from build123d import *

# Parameters (mm, degrees)
SKETCH1_R           = 74.5
BOSS_EXTRUDE1_DEPTH = 385.699
SKETCH2_W           = 27.8577878
SKETCH2_H           = 360.299
SKETCH3_R           = 4.499991
CUT_EXTRUDE1_DEPTH  = 400.830237227
CIRPATTERN1_COUNT   = 4
FILLET1_R           = 10


with BuildPart() as part:
    # Sketch1 → Boss-Extrude1 (new body)
    with BuildSketch(Plane(origin=(0, 0, 0), x_dir=(1, 0, 0), z_dir=(0, 1, 0))):
        with Locations(Location((0, 0, 0), (0, 0, 270))):
            Circle(SKETCH1_R)
    extrude(amount=BOSS_EXTRUDE1_DEPTH)

    # Sketch2 → Cut-Revolve4 (revolve, cut)
    with BuildSketch(Plane.XY, mode=Mode.PRIVATE) as cut_revolve4_sk:
        with Locations((-60.5711061, 192.8495)):
            Rectangle(SKETCH2_W, SKETCH2_H)
    revolve(cut_revolve4_sk.sketch.rotate(Axis((0, 385.699, 0), (0, -1, 0)), 270), axis=Axis((0, 385.699, 0), (0, -1, 0)), mode=Mode.SUBTRACT)

    # Sketch3 → Cut-Extrude1 (cut, through all)
    with BuildSketch(Plane.XZ):
        with Locations(Location((0, 66.000122, 0), (0, 0, 270))):
            Circle(SKETCH3_R)
    cut_extrude1 = extrude(amount=-CUT_EXTRUDE1_DEPTH, mode=Mode.SUBTRACT)

    # CirPattern1: Cut-Extrude1 ×4 about axis
    cirpattern1_axis = Axis((0, 0, 0), (0, 1, 0))
    for i in range(1, CIRPATTERN1_COUNT):
        add(cut_extrude1.rotate(cirpattern1_axis, i * 360 / CIRPATTERN1_COUNT), mode=Mode.SUBTRACT)

    # Fillet1
    fillet1_edges = [part.edges().sort_by_distance(p)[0] for p in [
        (0, 12.7, -46.6422122),
        (0, 372.999, -46.6422122),
    ]]
    fillet(fillet1_edges, radius=FILLET1_R)


solid = part.part
The listing builds one solid part. Answer for the finished solid, in the listing's coordinates (mm). A direction names the side the tool comes from. Coordinates: 2 decimals unless noted, no trailing zeros. Order: outer loops, then holes, each group sorted by start corner. A loop starts at its lowest first (then second) coordinate and runs counter-clockwise, first axis right, second up. Notation, with made-up numbers: (-8, 31) -> (-4, 31) arc R17 cw to (-4, 40) -> close; hole circle Ø10 at (76, -7). An arc over 180 degrees is marked (long way). Answer in a Markdown table with one row per item. Add a question column.
Item 1: Find section A-A (x = 0). State how many separate pieces and enclosed holes the cut face has, then the cut area to 3 significant figures.
Item 2: Find the intervals of material crossed by L1, parallel to Y at x = -39.5, z = -48; L2, parallel to Y at x = 17, z = 46; L3, parallel to X at y = 195.5, z = 24.5, in increasing order. Write a range as from..to.
Item 3: Each of these flat-tipped pins is pushed along its axis until it touches: P1, Ø8, axis at y = 90, z = 21.5, coming from the -X side; P2, Ø12, axis at y = 267.5, z = 28, coming from the -X side; P3, Ø4, axis at y = 271, z = -28.5, coming from the +X side. Where does it stop, or does it pass through?
Item 4: Which of the six approach directions +Z, -Z, +X, -X, +Y, -Y give full straight-line access (tool end or side, diameter ignored) to faces 1 (the face through (-70.496, 6.261, 0.198)), 2 (the face through (27, 372.999, -50))?
Item 5: Find section C-C (y = 154). Write down the section's boundary in (x, z), then the cut area to 3 significant figures.
Item 6: Determine the mould class of faces 3 (the face through (22.38, 6.26, 71.06)), 4 (the face through (-14.01, 195.23, 44.49)), 5 (the face through (1, 385.699, -1)) for opening direction Y: +Y half, -Y half, draft (parallel to the pull), parting line (faces both ways), or undercut.
Result set:
| question | item | result |
|---|---|---|
| 1 | separate pieces | 5 |
| 1 | enclosed holes | 0 |
| 1 | area | 37,000 mm² |
| 2 | L1 | y = 0..12.7, 373..385.7 |
| 2 | L2 | y = 0..16.2, 369.5..385.7 |
| 2 | L3 | x = -39.69..39.69 |
| 3 | P1 | stops at x = -43.23 |
| 3 | P2 | stops at x = -41.13 |
| 3 | P3 | stops at x = 38.38 |
| 4 | face 1 | +Y, -Y |
| 4 | face 2 | none |
| 5 | outline | circle Ø93.28 at (0, 0) |
| 5 | area | 6,830 mm² |
| 6 | face 3 | draft |
| 6 | face 4 | undercut |
| 6 | face 5 | +Y half |
